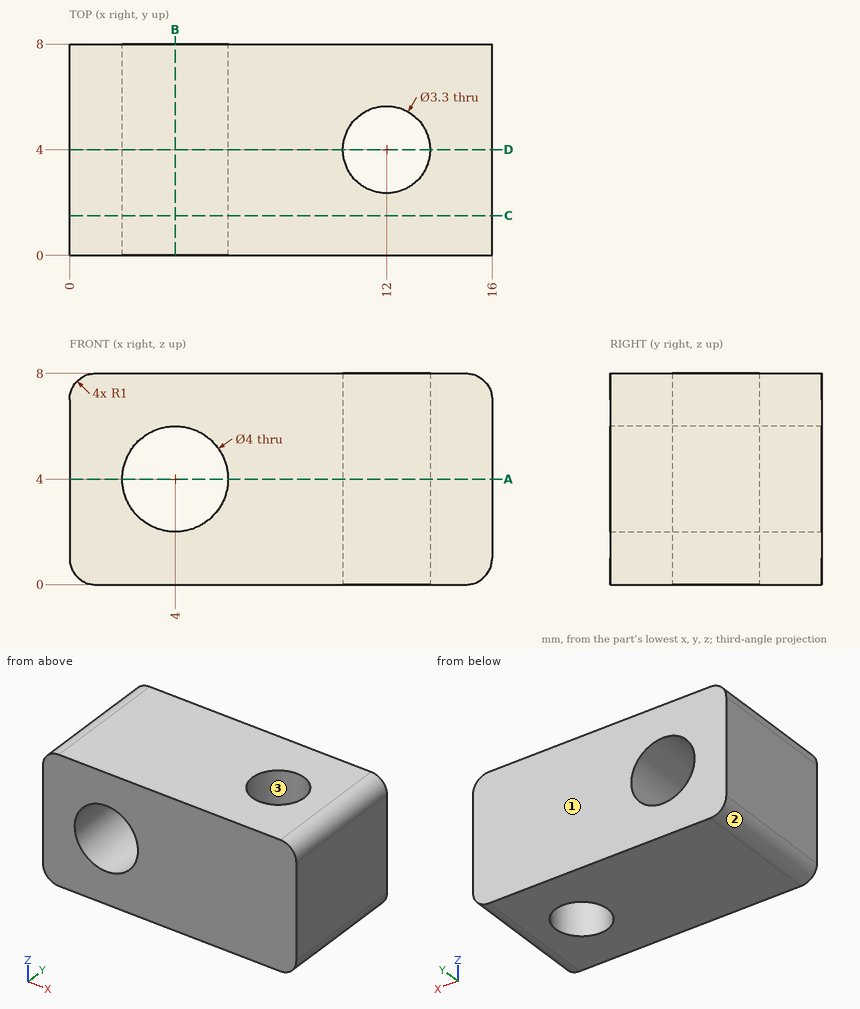
Can you work these out from the drawing? Everything is in mm from the part's minimum corner. Coordinates: 2 decimals unless noted, no trailing zeros. Loops run counter-clockwise (first coordinate to the right, second up) from the corner with the lowest first, then second, coordinate; pieces in that order, holes last. Notation, with made-up numbers: (46.25, 60) - (57.25, 60) arc R18 cw to (57.25, 78) - close; hole circle Ø4 at (7.25, 17.5). An arc over 180 degrees is marked (long way). Put each result on its own line as item: value. Start each with the question number.
Item 1: If we mould it in two halves opening along X, with no side actions, what happens to the marked faces 1, 2 and 3? For each: +X half, -X half, draft (parallel to the pull), parting line (faces both ways), or undercut.
Item 2: Suppose I cut it at A-A (z = 4). Please give me the cut outline in (x, y).
Item 3: If I drill on line 1 along X through (y, z) = (1, 4); line 2 along Y through (x, z) = (12, 5); line 3 along X through (y, z) = (5, 4), over which ranges is the centre line in solid material (lowest first)?
Item 4: Suppose I cut it at B-B (x = 4). Please give me the cut outline in (y, z).
Item 5: Suppose I cut it at D-D (y = 4). Please give me the cut outline in (x, z).
Item 6: Suppose I cut it at C-C (y = 1.5). Please give me the cut outline in (x, z).
Here are the results:
1. face 1: draft
1. face 2: -X half
1. face 3: undercut
2. outline: (0, 0) - (2, 0) - (2, 8) - (0, 8) - close; (6, 0) - (16, 0) - (16, 8) - (6, 8) - close; hole circle Ø3.3 at (12, 4)
3. line 1: 0 to 2, 6 to 16
3. line 2: 0 to 2.35, 5.65 to 8
3. line 3: 0 to 2, 6 to 10.69, 13.31 to 16
4. outline: (0, 0) - (8, 0) - (8, 2) - (0, 2) - close; (0, 6) - (8, 6) - (8, 8) - (0, 8) - close
5. outline: (0, 1) arc R1 ccw to (1, 0) - (10.35, 0) - (10.35, 8) - (1, 8) arc R1 ccw to (0, 7) - close; (13.65, 0) - (15, 0) arc R1 ccw to (16, 1) - (16, 7) arc R1 ccw to (15, 8) - (13.65, 8) - close; hole circle Ø4 at (4, 4)
6. outline: (0, 1) arc R1 ccw to (1, 0) - (15, 0) arc R1 ccw to (16, 1) - (16, 7) arc R1 ccw to (15, 8) - (1, 8) arc R1 ccw to (0, 7) - close; hole circle Ø4 at (4, 4)
